from build123d import *

# Parameters (mm, degrees)
BOSS_EXTRUDE1_DEPTH = 10


with BuildPart() as part:
    # Sketch4 → Boss-Extrude1 (new body)
    with BuildSketch(Plane.XY):
        with BuildLine():
            ThreePointArc((0.8, 0), (0.234314575, 0.234314575), (0, 0.8))
            Line((0, 0.8), (0, 21.2))
            ThreePointArc((0, 21.2), (0.234314575, 21.765685425), (0.8, 22))
            Line((0.8, 22), (6.2, 22))
            ThreePointArc((6.2, 22), (7.472792206, 21.472792206), (8, 20.2))
            Line((8, 20.2), (8, 20.15))
            Line((8, 20.15), (2.85, 20.15))
            Line((2.85, 20.15), (2.85, 10.15))
            Line((2.85, 10.15), (8, 10.15))
            Line((8, 10.15), (8, 10.1))
            ThreePointArc((8, 10.1), (7.472792206, 8.827207794), (6.2, 8.3))
            Line((6.2, 8.3), (5.8, 8.3))
            ThreePointArc((5.8, 8.3), (4.527207794, 7.772792206), (4, 6.5))
            Line((4, 6.5), (4, 2.8))
            ThreePointArc((4, 2.8), (3.179898987, 0.820101013), (1.2, 0))
            Line((1.2, 0), (0.8, 0))
        make_face()
        with BuildLine():
            ThreePointArc((4.663339973, 20.15), (5.5, 19.15), (6.336660027, 20.15))
            Line((6.336660027, 20.15), (4.663339973, 20.15))
        make_face()
        with BuildLine():
            Line((4.663339973, 10.15), (6.336660027, 10.15))
            ThreePointArc((6.336660027, 10.15), (5.5, 11.15), (4.663339973, 10.15))
        make_face()
    extrude(amount=BOSS_EXTRUDE1_DEPTH)


solid = part.part
Verification items for the finished model (mm, model axes). A direction names the side the tool comes from. Give positions to 0.01 mm unless a question says otherwise; leave off trailing zeros. Loops run counter-clockwise (first coordinate to the right, second up) from the corner with the lowest first, then second, coordinate; pieces in that order, holes last.
1. Tool access check on faces 5 (the flat face through (4, 5, 5)), 6 (the flat face through (2.85, 15, 5)), 7 (the flat face through (7, 10.15, 5)). Record the directions out of +Z, -Z, +X, -X, +Y, -Y that give a thin tool (end or side, any length) a straight path to the whole face; none if there is none.
Derived:
face 5: +Z, -Z, +X, -Y
face 6: +Z, -Z
face 7: +Z, -Z, +X
2. Release check for a two-part mould opening along Y. For faces 1 (the flat face through (3, 22, 5)), 2 (the flat face through (4, 20.15, 5)), 3 (the flat face through (0, 11, 5)), 4 (the flat face through (7, 20.15, 5)) record: +Y half, -Y half, draft (parallel to the pull), parting line (faces both ways), or undercut.
Derived:
face 1: +Y half
face 2: undercut
face 3: draft
face 4: undercut
3. Cross-section at C-C on y = 12.5. Record the cut outline in (x, z), and give its area (3 significant figures).
Derived:
outline: (0, 0) - (2.85, 0) - (2.85, 10) - (0, 10) - close
area: 28.5 mm2
4. Go/stop test with flat-tipped pins: P1, Ø0.9, axis at x = 3.5, z = 4.5, coming from the -Y side; P2, Ø0.8, axis at x = 7.5, z = 5, coming from the +Y side; P3, Ø1.8, axis at x = 7, z = 5.5, coming from the -Y side. Record where each tip stops, or that it passes through.
Derived:
P1: stops at y = 0.7
P2: stops at y = 21.76
P3: stops at y = 8.3
5. Cross-section at A-A on x = 5.5. Record the cut outline in (y, z).
Derived:
outline: (8.27, 0) - (11.15, 0) - (11.15, 10) - (8.27, 10) - close; (19.15, 0) - (22, 0) - (22, 10) - (19.15, 10) - close
6. Cross-section at D-D on x = 3.75. Record the cut outline in (y, z).
Derived:
outline: (1.64, 0) - (10.15, 0) - (10.15, 10) - (1.64, 10) - close; (20.15, 0) - (22, 0) - (22, 10) - (20.15, 10) - close
7. Material ranges on probe 1 along X at (y, z) = (13.25, 6); probe 2 along Y at (x, z) = (4.75, 4.25); probe 3 along Y at (x, z) = (5, 7.75), recorded low to high.
Derived:
probe 1: x = 0 to 2.85
probe 2: y = 7.96 to 10.7, 19.6 to 22
probe 3: y = 8.11 to 10.99, 19.31 to 22
8. Cross-section at B-B on z = 8. Record the cut outline in (x, y), and give its area (3 significant figures).
Derived:
outline: (0, 0.8) arc R0.8 ccw to (0.8, 0) - (1.2, 0) arc R2.8 ccw to (4, 2.8) - (4, 6.5) arc R1.8 cw to (5.8, 8.3) - (6.2, 8.3) arc R1.8 ccw to (8, 10.1) - (8, 10.15) - (6.34, 10.15) arc R0.85 ccw (long way) to (4.66, 10.15) - (2.85, 10.15) - (2.85, 20.15) - (4.66, 20.15) arc R0.85 ccw (long way) to (6.34, 20.15) - (8, 20.15) - (8, 20.2) arc R1.8 ccw to (6.2, 22) - (0.8, 22) arc R0.8 ccw to (0, 21.2) - close
area: 91.4 mm2
